```python
from build123d import *
from OCP.BRepAlgoAPI import BRepAlgoAPI_Cut
from OCP.TopTools import TopTools_ListOfShape

# Parameters (mm, degrees)
SKETCH1_R           = 10
SKETCH1_R_2         = 4.5
BOSS_EXTRUDE1_DEPTH = 2.776375223
SKETCH2_R           = 6
SKETCH2_R_2         = 4.5
BOSS_EXTRUDE3_DEPTH = 3.223625257
SKETCH3_R           = 6
SKETCH3_R_2         = 3.5
BOSS_EXTRUDE4_DEPTH = 3.45
SKETCH4_R           = 6
BOSS_EXTRUDE5_DEPTH = 9.75
SKETCH5_R           = 6
BOSS_EXTRUDE6_DEPTH = 0.6
CUT_EXTRUDE1_START  = -0.35
SKETCH6_R           = 10
SKETCH6_R_2         = 6
CUT_EXTRUDE1_DEPTH  = 0.35


with BuildPart() as part:
    # Sketch1 → Boss-Extrude1 (new body)
    with BuildSketch(Plane.XY.offset(1)):
        with Locations((-18.768000381, 45.999999683)):
            Circle(SKETCH1_R)
        with Locations((-18.768000381, 45.999999683)):
            Circle(SKETCH1_R_2, mode=Mode.SUBTRACT)
    extrude(amount=BOSS_EXTRUDE1_DEPTH)

    # Sketch2 → Boss-Extrude3 (add)
    with BuildSketch(Plane(origin=(-3.3e-07, 0, 3.77637599), x_dir=(0.9999999999999963, 0, 8.742277657347971e-08), z_dir=(-8.742277657347971e-08, -3.821370931908002e-15, 0.9999999999999963))):
        with Locations(Location((-18.76800005, 45.999999683, 0), (0, 0, 180))):
            Circle(SKETCH2_R)
        with Locations((-18.76800005, 45.999999683)):
            Circle(SKETCH2_R_2, mode=Mode.SUBTRACT)
    extrude(amount=BOSS_EXTRUDE3_DEPTH)


with BuildPart() as boss_extrude4_tool:
    # Sketch3 → Boss-Extrude4 (new body)
    with BuildSketch(Plane.XY.offset(7)):
        with Locations((-18.768000662, 45.999999683)):
            Circle(SKETCH3_R)
        with Locations((-18.768000381, 45.999999683)):
            Circle(SKETCH3_R_2, mode=Mode.SUBTRACT)
    extrude(amount=BOSS_EXTRUDE4_DEPTH)


with BuildPart() as part_1:
    add(part.part)


with BuildPart() as part_2:
    # Boss-Extrude4: joined with boss_extrude4_tool
    add(part_1.part.fuse(boss_extrude4_tool.part, tol=0.00001))

    # Sketch4 → Boss-Extrude5 (add)
    with BuildSketch(Plane.XY.offset(10.45)):
        with Locations((-18.768000662, 45.999999683)):
            Circle(SKETCH4_R)
        with BuildLine():
            Line((-17.100629081, 49.07731555), (-17.100628812, 42.922683961))
            ThreePointArc((-17.100628812, 42.922683961), (-22.268000381, 45.99999953), (-17.100629081, 49.07731555))
        make_face(mode=Mode.SUBTRACT)
    extrude(amount=BOSS_EXTRUDE5_DEPTH)

    # Sketch5 → Boss-Extrude6 (add)
    with BuildSketch(Plane.XY.offset(20.2)):
        with Locations((-18.768000662, 45.999999683)):
            Circle(SKETCH5_R)
    extrude(amount=BOSS_EXTRUDE6_DEPTH)


with BuildPart() as cut_extrude1_tool:
    # Sketch6 → Cut-Extrude1 (new body)
    with BuildSketch(Plane(origin=(-3.3e-07, 0, 3.77637599), x_dir=(0.9999999999999963, 0, 8.742277657347971e-08), z_dir=(-8.742277657347971e-08, -3.821370931908002e-15, 0.9999999999999963)).offset(CUT_EXTRUDE1_START)):
        with Locations((-18.76800005, 45.999999683)):
            Circle(SKETCH6_R)
        with Locations((-18.76800005, 45.999999683)):
            Circle(SKETCH6_R_2, mode=Mode.SUBTRACT)
    extrude(amount=CUT_EXTRUDE1_DEPTH)


with BuildPart() as part_3:
    add(part_2.part)

    # Cut-Extrude1: cut by cut_extrude1_tool, with a tolerance
    cut_extrude1_stock = TopTools_ListOfShape()
    cut_extrude1_stock.Append(part_3.part.wrapped)
    cut_extrude1_tools = TopTools_ListOfShape()
    cut_extrude1_tools.Append(cut_extrude1_tool.part.wrapped)
    cut_extrude1_cut = BRepAlgoAPI_Cut()
    cut_extrude1_cut.SetArguments(cut_extrude1_stock)
    cut_extrude1_cut.SetTools(cut_extrude1_tools)
    cut_extrude1_cut.SetFuzzyValue(0.00001)
    cut_extrude1_cut.Build()
    add(Compound.cast(cut_extrude1_cut.Shape()).solids(), mode=Mode.REPLACE)


solid = part_3.part
```
CAD build for the part. Positions are in the model's coordinates, mm. A direction names the side the tool comes from. Round coordinates to 2 decimals unless told otherwise and drop trailing zeros. Loops run counter-clockwise (first coordinate to the right, second up) from the corner with the lowest first, then second, coordinate; pieces in that order, holes last. Notation, with made-up numbers: (42.5, -24) - (61.5, -24) arc R34 ccw to (61.5, 12) - close; hole circle Ø2 at (-5, 34). An arc over 180 degrees is marked (long way). Return JSON: item names as keys, results as strings. Group by question number.
Q1. Two-plate mould, pull along Y, no slides. Class faces 4 (the face through (-20.07, 55.915, 2.196)), 5 (the face through (-16.7, 41.7, 1)), 6 (the face through (-19, 46, 20.2)): +Y half, -Y half, draft (parallel to the pull), parting line (faces both ways), or undercut.
Q2. Band-saw the part on B-B on y = 44.25. Give the cut face in (x, z).
Q3. Band-saw the part on A-A on z = 13.25. Give the cut face in (x, y).
Q4. Drill centre lines: line 1 along X through (y, z) = (46, 5.3); line 2 along X through (y, z) = (46, 7.8); line 3 along Y through (x, z) = (-18, 12). Where is each one in solid material? Low to high. Write a range as [from, to].
Q5. Band-saw the part on C-C on x = -11. Give the cut face in (y, z).
Q6. Tool access for faces 1 (the face through (-14, 42, 3.426)), 2 (the face through (-19, 46, 20.8)), 3 (the face through (-16, 43, 7)): list every direction of +Z, -Z, +X, -X, +Y, -Y with a clear straight run to the whole face (end or side of a thin tool).
Q7. Band-saw the part on D-D on z = 8. Give the cut face in (x, y).
Q8. Flat gauge pins, fed straight in: pin 1 Ø2 at (x, y) = (-16, 45) entering from -Z; pin 2 Ø8 at (x, z) = (-18.5, 12.5) entering from -Y; pin 3 Ø1 at (x, z) = (-18.5, 7) entering from +Y. Where does each tip first touch, or does it go through?
Solutions:
{
 "1": {"face 4": "parting line", "face 5": "draft", "face 6": "undercut"},
 "2": {"outline": "(-28.61, 1) - (-22.91, 1) - (-22.91, 7) - (-21.8, 7) - (-21.8, 20.2) - (-17.1, 20.2) - (-17.1, 10.45) - (-15.74, 10.45) - (-15.74, 7) - (-14.62, 7) - (-14.62, 1) - (-8.92, 1) - (-8.92, 3.43) - (-13.03, 3.43) - (-13.03, 20.8) - (-24.51, 20.8) - (-24.51, 3.43) - (-28.61, 3.43) - close"},
 "3": {"outline": "circle Ø12 at (-18.77, 46); hole (-17.1, 42.92) - (-17.1, 49.08) arc R3.5 ccw (long way) to start"},
 "4": {"line 1": "x = [-24.77, -23.27], [-14.27, -12.77]", "line 2": "x = [-24.77, -22.27], [-15.27, -12.77]", "line 3": "y = [40.05, 42.59], [49.41, 51.95]"},
 "5": {"outline": "(39.7, 1) - (52.3, 1) - (52.3, 3.43) - (39.7, 3.43) - close"},
 "6": {"face 1": "+Z", "face 2": "+Z, +X, -X, +Y, -Y", "face 3": "-Z"},
 "7": {"outline": "circle Ø12 at (-18.77, 46); hole circle Ø7 at (-18.77, 46)"},
 "8": {"pin 1": "stops at z = 7", "pin 2": "stops at y = 40", "pin 3": "stops at y = 52"}
}
